Source: three-view drawing plus pictorial views. Frame: mm from the lowest corner of the part. Coordinates: 2 decimals unless noted, no trailing zeros. Loops run counter-clockwise (first coordinate to the right, second up) from the corner with the lowest first, then second, coordinate; pieces in that order, holes last.
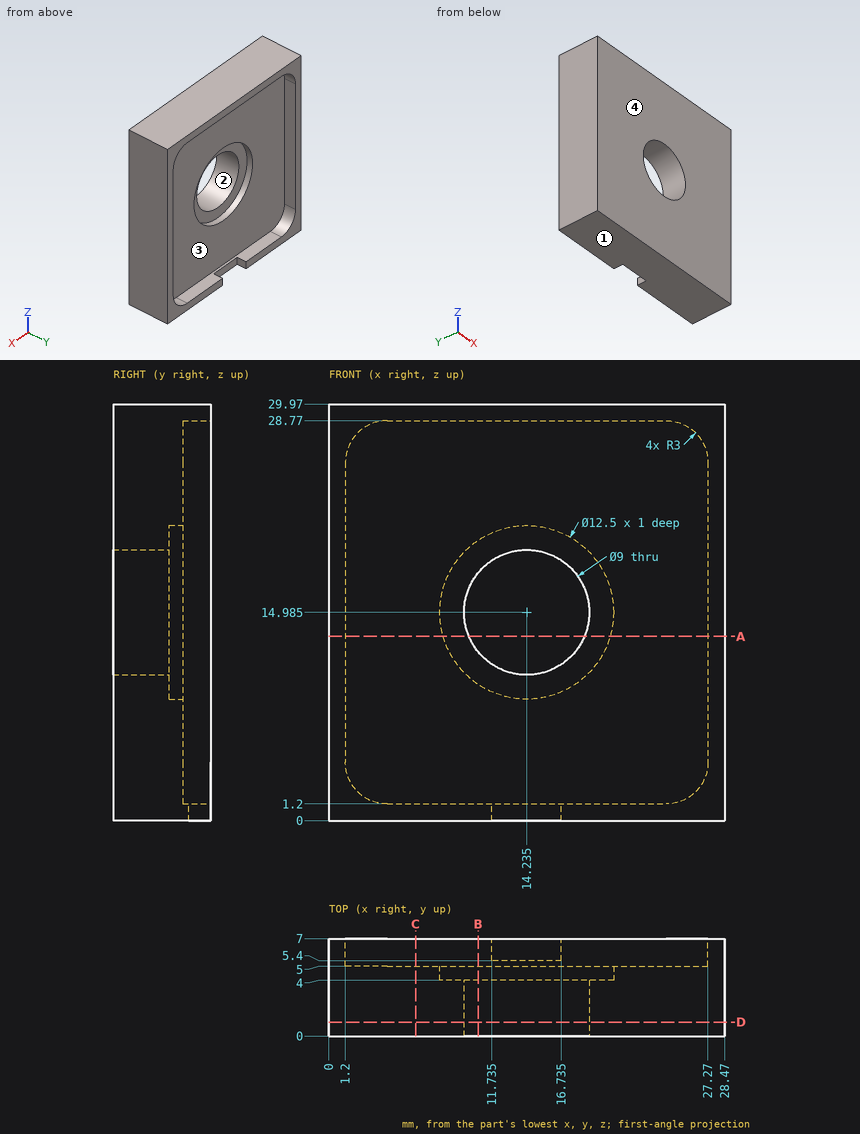
Q1. Section C-C, the plane x = 6.25. Return the cut outline in (y, z), plus the area to 3 significant figures.
Q2. Section B-B, the plane x = 10.75. Return the cut outline in (y, z), plus the area to 3 significant figures.
Q3. Section A-A, the plane z = 13.25. Return the cut outline in (x, y).
Q4. Section D-D, the plane y = 1. Return the cut outline in (x, z) (3 decimals).
Q5. Line query: line 1 along Z through (x, y) = (20.5, 6.5); line 2 along Y through (x, z) = (16.75, 7.75); line 3 along X through (y, z) = (6.5, 10). Output: solid intervals per line, ascending.
Q6. Draft query along Z for the marked faces 1, 2, 3 and 4. Return one class per face: +Z half, -Z half, draft (parallel to the pull), parting line (faces both ways), or undercut.
Q7. Contact query for flat-ended pins moving along their axis: pin 1 Ø8 at (x, z) = (18.5, 16) entering from +Y; pin 2 Ø4 at (x, z) = (15.5, 17.5) entering from +Y; pin 3 Ø7 at (x, z) = (14.235, 14.985) entering from +Y; pin 4 Ø1 at (x, y) = (15, 6) entering from -Z. Output: stop coordinate, or through.
Derived:
1. outline: (0, 0) - (7, 0) - (7, 1.2) - (5, 1.2) - (5, 28.77) - (7, 28.77) - (7, 29.97) - (0, 29.97) - close
1. area: 155 mm2
2. outline: (0, 0) - (7, 0) - (7, 1.2) - (5, 1.2) - (5, 9.8) - (4, 9.8) - (4, 12.14) - (0, 12.14) - close; (0, 17.83) - (4, 17.83) - (4, 20.17) - (5, 20.17) - (5, 28.77) - (7, 28.77) - (7, 29.97) - (0, 29.97) - close
2. area: 121 mm2
3. outline: (0, 0) - (10.08, 0) - (10.08, 4) - (8.23, 4) - (8.23, 5) - (1.2, 5) - (1.2, 7) - (0, 7) - close; (18.39, 0) - (28.47, 0) - (28.47, 7) - (27.27, 7) - (27.27, 5) - (20.24, 5) - (20.24, 4) - (18.39, 4) - close
4. outline: (0, 0) - (28.47, 0) - (28.47, 29.97) - (0, 29.97) - close; hole circle Ø9 at (14.235, 14.985)
5. line 1: z = 0 to 1.2, 28.77 to 29.97
5. line 2: y = 0 to 5
5. line 3: x = 0 to 1.2, 27.27 to 28.47
6. face 1: -Z half
6. face 2: undercut
6. face 3: undercut
6. face 4: draft
7. pin 1: stops at y = 5
7. pin 2: stops at y = 4
7. pin 3: passes through
7. pin 4: stops at z = 28.77
